Work out the finished part from the listing and answer in its coordinate system (mm). Face numbers are marked on the shaded views. A direction names the side the tool comes from. Give positions to 0.01 mm unless a question says otherwise; leave off trailing zeros. Loops run counter-clockwise (first coordinate to the right, second up) from the corner with the lowest first, then second, coordinate; pieces in that order, holes last. Notation, with made-up numbers: M -25.75,63 L 21.25,63 A11 cw 21.25,84 Z; hole C 73.25,8.25 d1. An arc over 180 degrees is marked long. Answer in a Markdown table with one row per item. Add a question column.
from build123d import *

# Parameters (mm, degrees)
F0_W          = 20
F0_H          = 20
F1_DEPTH      = 20
F2_D          = 3
F2_DEPTH      = 20
F2_TIP        = 0.9012909285
F3_D          = 16
F3_DEPTH      = 20
F3_TIP        = 4.8068849522
F4_W          = 40
F4_H          = 32
F4_R          = 1.5
F5_DEPTH      = 11.5
F7_D          = 2.5
F7_DEPTH      = 5
F7_TIP        = 0.7510757738
F8_R          = 5
F10_D         = 2.5
F10_DEPTH     = 5
F10_TIP       = 0.7510757738
F11_T1_DEPTH  = 22.5
F11_T3_DEPTH  = 55
F11_T5_DEPTH  = 30
F11_T8_ANGLE  = 90
F11_T10_ANGLE = 90
F13_W         = 5
F13_H         = 10
F14_DEPTH     = 25
F15_R         = 3
F16_D         = 2
F16_DEPTH     = 5
F16_TIP       = 0.600860619


# Not quite as in the source:
# - a fillet or chamfer that OpenCascade refuses, or shapes differently, is made with other operations: its cross-section is extruded or revolved along the edge and cut away or added


with BuildPart() as f1:
    # F0 (on Top) → F1 (new body)
    with BuildSketch(Plane.XY):
        with Locations((-5, 20)):
            Rectangle(F0_W, F0_H)
        with Locations((15, 20)):
            Rectangle(F0_W, F0_H)
        Polygon((5, 10), (-15, 10), (-15, -22), (25, -22), (25, 10), align=None)
    extrude(amount=-F1_DEPTH)

    # F2
    with Locations(Plane.XY):
        with Locations((10, 0), (0, 0), (0, -12), (10, -12)):
            Hole(F2_D / 2, depth=F2_DEPTH)
            with Locations((0, 0, -(F2_DEPTH + F2_TIP / 2))):  # 118° drill point
                Cone(0, F2_D / 2, F2_TIP, mode=Mode.SUBTRACT)

    # F3
    with Locations(Plane.XY):
        with Locations((15, 20), (-5, 20)):
            Hole(F3_D / 2, depth=F3_DEPTH)
            with Locations((0, 0, -(F3_DEPTH + F3_TIP / 2))):  # 118° drill point
                Cone(0, F3_D / 2, F3_TIP, mode=Mode.SUBTRACT)

    # F4 (on face) → F5 (cut)
    with BuildSketch(Plane(origin=(0, 0, -20), x_dir=(1, 0, 0), z_dir=(0, 0, -1))):
        with Locations((5, 6)):
            Rectangle(F4_W, F4_H)
        Circle(F4_R, mode=Mode.SUBTRACT)
        with Locations((0, 12)):
            Circle(F4_R, mode=Mode.SUBTRACT)
        with Locations((10, 0)):
            Circle(F4_R, mode=Mode.SUBTRACT)
        with Locations((10, 12)):
            Circle(F4_R, mode=Mode.SUBTRACT)
    extrude(amount=-F5_DEPTH, mode=Mode.SUBTRACT)

    # F7
    with Locations(Plane.XZ.offset(22)):
        with Locations((-5, -4.25), (15, -4.25)):
            Hole(F7_D / 2, depth=F7_DEPTH)
            with Locations((0, 0, -(F7_DEPTH + F7_TIP / 2))):  # 118° drill point
                Cone(0, F7_D / 2, F7_TIP, mode=Mode.SUBTRACT)

    # F8
    f8_edges = [f1.edges().sort_by_distance(p)[0] for p in [
        (-15, 30, -10),
        (25, 30, -10),
    ]]
    fillet(f8_edges, radius=F8_R)

    # F10
    with Locations(Plane(origin=(0, 30, 0), x_dir=(-1, 0, 0), z_dir=(0, 1, 0))):
        with Locations((5, -10), (-15, -10)):
            Hole(F10_D / 2, depth=F10_DEPTH)
            with Locations((0, 0, -(F10_DEPTH + F10_TIP / 2))):  # 118° drill point
                Cone(0, F10_D / 2, F10_TIP, mode=Mode.SUBTRACT)

    # F11: fillet of radius 3 on 2 edges, made by hand

    # F11_s2 → F11_t1 (cut)
    with BuildSketch(Plane.XZ.offset(-25)):
        with BuildLine():
            ThreePointArc((-15, -17), (-14.1213203436, -19.1213203436), (-12, -20))
            Line((-12, -20), (-15, -20))
            Line((-15, -20), (-15, -17))
        make_face()
        with BuildLine():
            ThreePointArc((22, -20), (24.1213203436, -19.1213203436), (25, -17))
            Line((25, -17), (25, -20))
            Line((25, -20), (22, -20))
        make_face()
    extrude(amount=F11_T1_DEPTH, mode=Mode.SUBTRACT)

    # F11_s4 → F11_t3 (cut)
    with BuildSketch(Plane.YZ.offset(-22.5)):
        with BuildLine():
            ThreePointArc((13, -20), (10.8786796564, -19.1213203436), (10, -17))
            Line((10, -17), (10, -20))
            Line((10, -20), (13, -20))
        make_face()
    extrude(amount=F11_T3_DEPTH, mode=Mode.SUBTRACT)

    # F11_s6 → F11_t5 (cut)
    with BuildSketch(Plane.YZ.offset(-10)):
        with BuildLine():
            ThreePointArc((27, -20), (29.1213203436, -19.1213203436), (30, -17))
            Line((30, -17), (30, -20))
            Line((30, -20), (27, -20))
        make_face()
    extrude(amount=F11_T5_DEPTH, mode=Mode.SUBTRACT)

    # F11_s7 → F11_t8 (revolve, cut)
    with BuildSketch(Plane.XZ.offset(-25)):
        with BuildLine():
            ThreePointArc((-15, -17), (-14.1213203436, -19.1213203436), (-12, -20))
            Line((-12, -20), (-15, -20))
            Line((-15, -20), (-15, -17))
        make_face()
    revolve(axis=Axis((-10, 25, -20), (0, 0, -1)), revolution_arc=F11_T8_ANGLE, mode=Mode.SUBTRACT)

    # F11_s9 → F11_t10 (revolve, cut)
    with BuildSketch(Plane.YZ.offset(20)):
        with BuildLine():
            ThreePointArc((27, -20), (29.1213203436, -19.1213203436), (30, -17))
            Line((30, -17), (30, -20))
            Line((30, -20), (27, -20))
        make_face()
    revolve(axis=Axis((20, 25, -20), (0, 0, -1)), revolution_arc=F11_T10_ANGLE, mode=Mode.SUBTRACT)

    # F13 (on face) → F14 (cut)
    with BuildSketch(Plane.XY):
        with Locations((22.5, 5)):
            Rectangle(F13_W, F13_H)
    extrude(amount=-F14_DEPTH, mode=Mode.SUBTRACT)

    # F15
    f15_edges = [f1.edges().sort_by_distance(p)[0] for p in [
        (20, 10, -4.25),
        (20, 0, -4.25),
    ]]
    fillet(f15_edges, radius=F15_R)

    # F16
    with Locations(Plane.YZ.offset(25)):
        with Locations((-13.5, -4.25), (11.5, -4.25)):
            Hole(F16_D / 2, depth=F16_DEPTH)
            with Locations((0, 0, -(F16_DEPTH + F16_TIP / 2))):  # 118° drill point
                Cone(0, F16_D / 2, F16_TIP, mode=Mode.SUBTRACT)


solid = f1.part
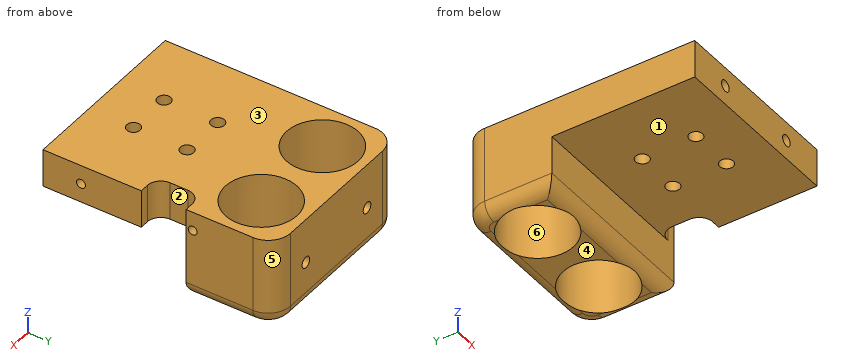
(1) Section D-D, the plane y = 15.5 is taken. Determine the outline of the cut face in (x, z), and give its area (3 significant figures).
(2) Which of the six approach directions +Z, -Z, +X, -X, +Y, -Y give full straight-line access (tool end or side, diameter ignored) to the marked faces 1, 2 and 3?
(3) Consider line 1 along X through (y, z) = (-12, -4.5); line 2 along X through (y, z) = (17, -4); line 3 along Y through (x, z) = (15, -1.5). Determine where each line is inside the solid, lowest interval first. Write a range as from..to.
(4) Each of these flat-tipped pins is pushed along its axis until it touches: P1, Ø8, axis at x = 8, z = -14.5, coming from the -Y side; P2, Ø1.6, axis at x = 24, z = -2.5, coming from the +Y side; P3, Ø9.5, axis at x = -4.5, y = -6.5, coming from the -Z side. Where does it stop, or does it pass through?
(5) Section B-B, the plane x = 0 is taken. Determine the outline of the cut face in (y, z) (3 decimals).
(6) Section A-A, the plane y = 21.5 is taken. Determine the outline of the cut face in (x, z), and give its area (3 significant figures).
(7) Section C-C, the plane x = 6 is taken. Determine the outline of the cut face in (y, z).
(8) The mould has two halves that part along Y. Classify the marked faces 4, 5 and 6: pulls with the +Y half, pulls with the -Y half, needs draft (parallel to the pull), parting line crosses it, or undercut.
Numbers:
| question | item | result |
|---|---|---|
| 1 | outline | M -15,-17 A3 ccw -12,-20 L -11.61,-20 L -11.61,0 L -15,0 Z; M 1.61,-20 L 8.39,-20 L 8.39,0 L 1.61,0 Z; M 21.61,-20 L 22,-20 A3 ccw 25,-17 L 25,0 L 21.61,0 Z |
| 1 | area | 267 mm² |
| 2 | face 1 | -Z, +X, -X, -Y |
| 2 | face 2 | +Z, -Z, +X |
| 2 | face 3 | +Z, +X, -X, +Y, -Y |
| 3 | line 1 | x = -15..-1.5, 1.5..8.5, 11.5..25 |
| 3 | line 2 | x = -15..-12.42, 2.42..7.58, 22.42..25 |
| 3 | line 3 | y = -22..12, 28..30 |
| 4 | P1 | stops at y = 10 |
| 4 | P2 | stops at y = 28.84 |
| 4 | P3 | stops at z = -8.5 |
| 5 | outline | M -22,-8.5 L -13.5,-8.5 L -13.5,0 L -22,0 Z; M -10.5,-8.5 L -1.5,-8.5 L -1.5,0 L -10.5,0 Z; M 1.5,-8.5 L 10,-8.5 L 10,-17 A3 ccw 13,-20 L 13.755,-20 L 13.755,0 L 1.5,0 Z; M 26.245,-20 L 27,-20 A3 ccw 30,-17 L 30,0 L 26.245,0 Z |
| 6 | outline | M -15,-17 A3 ccw -12.86,-19.87 L -12.86,0 L -15,0 Z; M 2.86,-20 L 7.14,-20 L 7.14,0 L 2.86,0 Z; M 22.86,-19.87 A3 ccw 25,-17 L 25,0 L 22.86,0 Z |
| 6 | area | 168 mm² |
| 7 | outline | M -22,-8.5 L 10,-8.5 L 10,-17 A3 ccw 13,-20 L 27,-20 A3 ccw 30,-17 L 30,0 L -22,0 Z |
| 8 | face 4 | needs draft |
| 8 | face 5 | pulls with the +Y half |
| 8 | face 6 | undercut |
